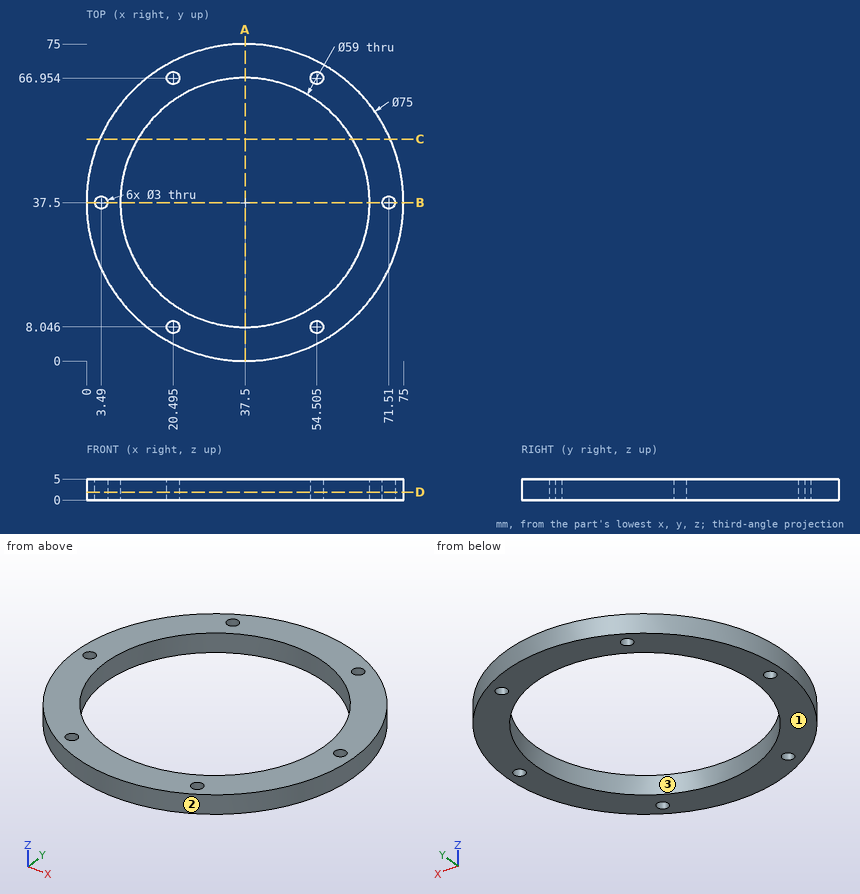
Can you work these out from the drawing? Everything is in mm from the part's minimum corner. Give positions to 0.01 mm unless a question says otherwise; leave off trailing zeros. Order: outer loops, then holes, each group sorted by start corner. A loop starts at its lowest first (then second) coordinate and runs counter-clockwise, first axis right, second up.
1. Will these pins go through, and if not, where does the flat tip stop? P1, Ø5, axis at x = 54.5, y = 66.95, coming from the +Z side; P2, Ø1, axis at y = 45.5, z = 1, coming from the +X side; P3, Ø1.5, axis at y = 40.5, z = 0.5, coming from the +X side; P4, Ø3, axis at x = 66.5, z = 3.5, coming from the +Y side (1 decimal).
2. Suppose I cut it at B-B (y = 37.5). List the corners of the cut face in (x, z) for me.
3. Suppose I cut it at D-D (z = 1.9). List the corners of the cut face in (x, y) for me (1 decimal), plus the area to 3 significant figures.
4. Suppose I cut it at C-C (y = 52.5). List the corners of the cut face in (x, z) for me.
5. We'd pull the mould along Y, two halves only. Please class the marked faces 1, 2 and 3: pulls with the +Y half, pulls with the -Y half, needs draft (parallel to the pull), parting line crosses it, or undercut.
6. Suppose I cut it at A-A (x = 37.5). List the corners of the cut face in (y, z) for me.
7. I need wall thicknesses on L1, parallel to X at y = 37, z = 0.8 (1 decimal); L2, parallel to Y at x = 37.5, z = 3.4; L3, parallel to X at y = 47.5, z = 2.5 (1 decimal). Which ranges of each line are inside material? Lowest first, please.
Solved:
1. P1: stops at z = 5
1. P2: stops at x = 74.24
1. P3: stops at x = 74.93
1. P4: stops at y = 63
2. outline: (0, 0) - (1.99, 0) - (1.99, 5) - (0, 5) - close; (4.99, 0) - (8, 0) - (8, 5) - (4.99, 5) - close; (67, 0) - (70.01, 0) - (70.01, 5) - (67, 5) - close; (73.01, 0) - (75, 0) - (75, 5) - (73.01, 5) - close
3. outline: circle Ø75 at (37.5, 37.5); hole circle Ø3 at (3.5, 37.5); hole circle Ø59 at (37.5, 37.5); hole circle Ø3 at (20.5, 8); hole circle Ø3 at (20.5, 67); hole circle Ø3 at (54.5, 8); hole circle Ø3 at (54.5, 67); hole circle Ø3 at (71.5, 37.5)
3. area: 1,640 mm2
4. outline: (3.13, 0) - (12.1, 0) - (12.1, 5) - (3.13, 5) - close; (62.9, 0) - (71.87, 0) - (71.87, 5) - (62.9, 5) - close
5. face 1: needs draft
5. face 2: parting line crosses it
5. face 3: undercut
6. outline: (0, 0) - (8, 0) - (8, 5) - (0, 5) - close; (67, 0) - (75, 0) - (75, 5) - (67, 5) - close
7. L1: x = 0 to 2.1, 4.9 to 8, 67 to 70.1, 72.9 to 75
7. L2: y = 0 to 8, 67 to 75
7. L3: x = 1.4 to 9.7, 65.3 to 73.6
